Geometry check sheet. Reference: the model listing, model coordinates, mm. A direction names the side the tool comes from. Coordinates: 2 decimals unless noted, no trailing zeros. Loops run counter-clockwise (first coordinate to the right, second up) from the corner with the lowest first, then second, coordinate; pieces in that order, holes last. Notation, with made-up numbers: M 85,-26 L 114,-26 A13 cw 114,-5 Z; hole C 9,-24 d4. An arc over 180 degrees is marked long. Use CSV: the item, a comma, the result in double quotes.
```python
from build123d import *

# Parameters (mm, degrees)
BOSS_EXTRUDE1_OUTLINE_R = 1.5
BOSS_EXTRUDE1_DEPTH     = 3
SKETCH1_R               = 1.5
CUT_EXTRUDE1_DEPTH      = 10
CIRPATTERN1_COUNT       = 4
SKETCH3_W               = 736.909485963
SKETCH3_H               = 680.360125743
CUT_EXTRUDE2_DEPTH      = 304.313928241
FILLET2_R               = 5
FILLET3_R               = 5
SKETCH4_R               = 1.5
CUT_EXTRUDE3_DEPTH      = 10


# Read off the part's stored shape, not the designer's step: Boss-Extrude1
with BuildPart() as part:
    # Boss-Extrude1 outline → Boss-Extrude1 (new body)
    with BuildSketch(Plane.XY):
        with BuildLine():
            ThreePointArc((227.170370868, 138.011217036), (227.042775693, 138.652681301), (227, 139.305312262))
            Line((227, 139.305312262), (227, 176.497490519))
            ThreePointArc((227, 176.497490519), (225.535533906, 180.033024425), (222, 181.497490519))
            Line((222, 181.497490519), (12.343347406, 181.497486855))
            ThreePointArc((12.343347406, 181.497486855), (8.909508183, 179.979649569), (7.5, 176.499941461))
            Line((7.5, 176.499941461), (7.5, 130.6))
            ThreePointArc((7.5, 130.6), (6.035533906, 127.064466094), (2.5, 125.6))
            Line((2.5, 125.6), (-4, 125.6))
            ThreePointArc((-4, 125.6), (-7.535533906, 124.135533906), (-9, 120.6))
            Line((-9, 120.6), (-9, 23.4))
            ThreePointArc((-9, 23.4), (-7.535533906, 19.864466094), (-4, 18.4))
            Line((-4, 18.4), (2.5, 18.4))
            ThreePointArc((2.5, 18.4), (6.035533906, 16.935533906), (7.5, 13.4))
            Line((7.5, 13.4), (7.5, -32.5))
            ThreePointArc((7.5, -32.5), (8.964466094, -36.035533906), (12.5, -37.5))
            Line((12.5, -37.5), (221.5, -37.5))
            ThreePointArc((221.5, -37.5), (225.035533906, -36.035533906), (226.5, -32.5))
            Line((226.5, -32.5), (226.5, 2.762899187))
            ThreePointArc((226.5, 2.762899187), (226.542775693, 3.415530148), (226.670370869, 4.056994413))
            Line((226.670370869, 4.056994413), (242.829629131, 64.364167262))
            ThreePointArc((242.829629131, 64.364167262), (242.957224307, 65.005631527), (243, 65.658262488))
            Line((243, 65.658262488), (243, 78.275974364))
            ThreePointArc((243, 78.275974364), (242.957224307, 78.928605325), (242.829629131, 79.570069589))
            Line((242.829629131, 79.570069589), (227.170370868, 138.011217036))
        make_face()
        with Locations((-2, 25.4)):
            Circle(BOSS_EXTRUDE1_OUTLINE_R, mode=Mode.SUBTRACT)
        with Locations((-2, 118.6)):
            Circle(BOSS_EXTRUDE1_OUTLINE_R, mode=Mode.SUBTRACT)
        with BuildLine():
            ThreePointArc((62.5, 68), (55.428932188, 65.071067812), (52.5, 58))
            Line((52.5, 58), (52.5, 52))
            ThreePointArc((52.5, 52), (51.035533906, 48.464466094), (47.5, 47))
            Line((47.5, 47), (12.5, 47))
            ThreePointArc((12.5, 47), (8.964466094, 48.464466094), (7.5, 52))
            Line((7.5, 52), (7.5, 92))
            ThreePointArc((7.5, 92), (8.964466094, 95.535533906), (12.5, 97))
            Line((12.5, 97), (47.5, 97))
            ThreePointArc((47.5, 97), (51.035533906, 95.535533906), (52.5, 92))
            Line((52.5, 92), (52.5, 86))
            ThreePointArc((52.5, 86), (55.428932188, 78.928932188), (62.5, 76))
            Line((62.5, 76), (117, 76))
            ThreePointArc((117, 76), (121, 72), (117, 68))
            Line((117, 68), (62.5, 68))
        make_face(mode=Mode.SUBTRACT)
        with Locations((236, 72)):
            Circle(BOSS_EXTRUDE1_OUTLINE_R, mode=Mode.SUBTRACT)
    extrude(amount=BOSS_EXTRUDE1_DEPTH)

    # Sketch1 → Cut-Extrude1 (cut)
    with BuildSketch(Plane.XY.offset(3)):
        with Locations((221.5, -32.501254741)):
            Circle(SKETCH1_R)
    cut_extrude1 = extrude(amount=-CUT_EXTRUDE1_DEPTH, mode=Mode.SUBTRACT)

    # CirPattern1: Cut-Extrude1 ×4 about axis
    cirpattern1_axis = Axis((117, 72, 0), (0, 0, 1))
    for i in range(1, CIRPATTERN1_COUNT):
        add(cut_extrude1.rotate(cirpattern1_axis, i * 360 / CIRPATTERN1_COUNT), mode=Mode.SUBTRACT)

    # Sketch3 → Cut-Extrude2 (cut, through all)
    with BuildSketch(Plane.XY.offset(3)):
        with Locations((306.942195916, -80.480880195)):
            Rectangle(SKETCH3_W, SKETCH3_H)
        Polygon((-4, 18.4), (10.001254741, 18.4), (10.001254741, -35), (224.001254741, -35), (224.001254741, -5.904282588), (241.995428238, 61.250887144), (247.405063047, 62.49431775), (224.001254741, 149.838519439), (224.001254741, 179), (10.001254741, 179), (10.001254741, 125.6), (-4, 125.6), (-27.04848394, 125.6), (-22.601157645, 14.939042157), align=None, mode=Mode.SUBTRACT)
    extrude(amount=-CUT_EXTRUDE2_DEPTH, mode=Mode.SUBTRACT)

    # Fillet2
    fillet2_edges = [part.edges().sort_by_distance(p)[0] for p in [
        (10.001254741, 125.6, 1.5),
        (10.001254741, 18.4, 1.5),
    ]]
    fillet(fillet2_edges, radius=FILLET2_R)

    # Fillet3
    fillet3_edges = [part.edges().sort_by_distance(p)[0] for p in [
        (224.001254741, -5.904282588, 1.5),
        (224.001254741, 149.838519439, 1.5),
    ]]
    fillet(fillet3_edges, radius=FILLET3_R)

    # Sketch4 → Cut-Extrude3 (cut)
    with BuildSketch(Plane(origin=(0, 0, 0), x_dir=(-1, 0, 0), z_dir=(0, 0, -1))):
        with Locations((2, 105.6)):
            Circle(SKETCH4_R)
        with Locations((2, 38.4)):
            Circle(SKETCH4_R)
    extrude(amount=-CUT_EXTRUDE3_DEPTH, mode=Mode.SUBTRACT)


solid = part.part
```
1. Release check for a two-part mould opening along Y. For faces 1 (the flat face through (115, 97, 0)), 2 (the cylindrical face through (55.35, 79.01, 1.48)), 3 (the cylindrical face through (8.575, 16.896, 1.479)) record: +Y half, -Y half, draft (parallel to the pull), parting line (faces both ways), or undercut.
The answers:
face 1,"draft"
face 2,"undercut"
face 3,"-Y half"
2. Gauge pin test, flat ends, axial feed: P1, Ø0.9, axis at y = -5.5, z = 2, coming from the -X side; P2, Ø1, axis at y = 118, z = 2, coming from the +X side; P3, Ø1.5, axis at y = 159, z = 1.5, coming from the +X side. Record the tip position at first contact, or that the pin passes through.
The answers:
P1,"x = 10"
P2,"x = 232.67"
P3,"x = 224"
3. Section check B-B, the plane x = 88. Record the cut outline in (y, z).
The answers:
outline,"M -35,0 L 68,0 L 68,3 L -35,3 Z; M 76,0 L 179,0 L 179,3 L 76,3 Z"
4. Section check A-A, the plane x = 20. Record the cut outline in (y, z).
The answers:
outline,"M -35,0 L 47,0 L 47,3 L -35,3 Z; M 97,0 L 179,0 L 179,3 L 97,3 Z"
5. Set-up check for faces 4 (the cylindrical face through (-7.57, 19.9, 1.48)), 5 (the cylindrical face through (51.07, 48.5, 1.48)): record each of +Z, -Z, +X, -X, +Y, -Y from which the full face is reachable in a straight line by a thin tool's end or side.
The answers:
face 4,"+Z, -Z, -X, -Y"
face 5,"+Z, -Z"
6. Thickness scan on line 1 (Y direction, x = -2, z = 1.9); line 2 (X direction, y = 72, z = 0.9); line 3 (X direction, y = -32.5, z = 1). Record the ranges inside material, lowest first. Write a range as [from, to].
The answers:
line 1,"[18.4, 23.9], [26.9, 36.9], [39.9, 104.1], [107.1, 117.1], [120.1, 125.6]"
line 2,"[-9, 7.5], [121, 234.5], [237.5, 243]"
line 3,"[10, 11], [14, 220], [223, 224]"
7. Section check C-C, the plane z = 2.1. Count the separate pieces of the cut face and the enclosed holes in it, plus the area to 3 significant figures.
The answers:
separate pieces,"1"
enclosed holes,"10"
area,"46,600 mm^2"
